Can you work these out from the model? Positions are in its coordinate system, mm. A direction names the side the tool comes from. Give positions to 0.01 mm unless a question says otherwise; leave off trailing zeros. Write each loop counter-clockwise with the first axis right and the second up, starting at its lowest first coordinate (ties: lowest second). Pieces come first, ordered by that corner, then holes. Notation, with made-up numbers: (57, 33) - (101, 33) arc R28 cw to (101, 70) - close; hole circle Ø5 at (53, 60). An arc over 180 degrees is marked (long way). Use a Markdown table: item, result. Add a question column.
```python
from build123d import *

# Parameters (mm, degrees)
F0_W     = 300
F0_H     = 50
F0_W_2   = 20
F1_DEPTH = 300
F2_W     = 50
F2_H     = 50
F3_DEPTH = 50
F4_DEPTH = 50


with BuildPart() as f1:
    # F0 (on Front) → F1 (new body)
    with BuildSketch(Plane.XZ):
        with Locations((-181.567696, 47.222274)):
            Rectangle(F0_W, F0_H)
        with Locations((-21.567696, 47.222274)):
            Rectangle(F0_W_2, F0_H)
        with Locations((138.432304, 47.222274)):
            Rectangle(F0_W, F0_H)
    extrude(amount=F1_DEPTH)

    # F2 (on face) → F3 (cut)
    with BuildSketch(Plane.XY.offset(72.222274)):
        with Locations((-306.567696, -150)):
            Rectangle(F2_W, F2_H)
        with Locations((263.432304, -150)):
            Rectangle(F2_W, F2_H)
    extrude(amount=-F3_DEPTH, mode=Mode.SUBTRACT)

    # F2 (on face) → F4 (cut)
    with BuildSketch(Plane.XY.offset(72.222274)):
        Polygon((-21.567696, -300), (-9.067696, -300), (-9.067696, -150), (-34.067696, -150), (-34.067696, -300), align=None)
    extrude(amount=-F4_DEPTH, mode=Mode.SUBTRACT)


solid = f1.part
```
Q1. Suppose I cut it at C-C (z = 43). Please give me the cut outline in (x, y).
Q2. I'm going to push flat-ended pins straight in: P1, Ø15, axis at y = -152, z = 54.5, coming from the -X side; P2, Ø15, axis at y = -160, z = 44, coming from the +X side. Where does each tip first touch, or does it pass through?
Q3. Suppose I cut it at A-A (y = -207.5). Please give me the cut outline in (x, z).
Q4. Suppose I cut it at B-B (x = 250.5). Please give me the cut outline in (y, z), and give its area (3 significant figures).
Q5. Suppose I cut it at D-D (y = -142.5). Please give me the cut outline in (x, z).
Q6. If we mould it in two halves opening along Y, with no side actions, what happens to faces 4 (the flat face through (-26, 0, 48)), 5 (the flat face through (263, -125, 48)), 6 (the flat face through (-331.568, -62, 47)), 7 (the flat face through (138, -300, 48))? For each: released by +Y, released by -Y, zero draft, split by the parting line, or undercut.
Q7. If I drill on probe 1 along X at (y, z) = (-209.5, 46.5); probe 2 along X at (y, z) = (-125.5, 69), over which ranges is the centre line in solid material (lowest first)? Write a range as [from, to].
Q8. On a 3-axis mill with a long thin cutter (end or side, diameter ignored), from which of +Z, -Z, +X, -X, +Y, -Y can I reach the whole of each face in a straight line? I mean faces 1 (the flat face through (-307, -125, 48)), 2 (the flat face through (-9.068, -226, 48)), 3 (the flat face through (238.432, -150, 48)). Say none if no direction works.
Derived:
| question | item | result |
|---|---|---|
| 1 | outline | (-331.57, -300) - (-34.07, -300) - (-34.07, -150) - (-9.07, -150) - (-9.07, -300) - (288.43, -300) - (288.43, -175) - (238.43, -175) - (238.43, -125) - (288.43, -125) - (288.43, 0) - (-331.57, 0) - (-331.57, -125) - (-281.57, -125) - (-281.57, -175) - (-331.57, -175) - close |
| 2 | P1 | x = -281.57 |
| 2 | P2 | x = 238.43 |
| 3 | outline | (-331.57, 22.22) - (-34.07, 22.22) - (-34.07, 72.22) - (-331.57, 72.22) - close; (-9.07, 22.22) - (288.43, 22.22) - (288.43, 72.22) - (-9.07, 72.22) - close |
| 4 | outline | (-300, 22.22) - (-175, 22.22) - (-175, 72.22) - (-300, 72.22) - close; (-125, 22.22) - (0, 22.22) - (0, 72.22) - (-125, 72.22) - close |
| 4 | area | 12,500 mm² |
| 5 | outline | (-281.57, 22.22) - (238.43, 22.22) - (238.43, 72.22) - (-281.57, 72.22) - close |
| 6 | face 4 | released by +Y |
| 6 | face 5 | undercut |
| 6 | face 6 | zero draft |
| 6 | face 7 | released by -Y |
| 7 | probe 1 | [-331.57, -34.07], [-9.07, 288.43] |
| 7 | probe 2 | [-281.57, 238.43] |
| 8 | face 1 | +Z, -Z, -X |
| 8 | face 2 | +Z, -Z, -Y |
| 8 | face 3 | +Z, -Z, +X |
